The model under review builds one solid part; all positions refer to its coordinate system, in mm. Face numbers are marked on the shaded views. A direction names the side the tool comes from. Give positions to 0.01 mm unless a question says otherwise; leave off trailing zeros. Loops run counter-clockwise (first coordinate to the right, second up) from the corner with the lowest first, then second, coordinate; pieces in that order, holes last. Notation, with made-up numbers: (-35.75, -16) -> (-2.75, -16) arc R19 ccw to (-2.75, 10) -> close; hole circle Ø1 at (5, 57.25). An arc over 180 degrees is marked (long way). Write each question's results on one line, items separated by ' | '. Start each with the question number.
Q1. We need section A-A (z = 20.25). Give the number of separate pieces and of enclosed holes in the cut face, plus the area to 4 significant figures.
Q2. Wall thickness on L1, parallel to Z at x = -28.5, y = -2.5; L2, parallel to X at y = -32, z = 19; L3, parallel to Y at x = 28.5, z = 4: over which ranges is each line inside the solid? List them lowest first. Write a range as [from, to].
Q3. Machinability: for the marked faces 1 and 2, which of the approach directions +Z, -Z, +X, -X, +Y, -Y give a long, thin tool a straight path to every point of the face, cutting with its end or side? Answer none if there is none.
Q4. Insertion check: pin 1 Ø1.3 at (x, z) = (15.5, 12.5) entering from +Y; pin 2 Ø8 at (y, z) = (-31.5, 9.5) entering from -X; pin 3 Ø8 at (x, z) = (-31.5, 9) entering from -Y; pin 4 Ø3 at (x, z) = (-32.5, 19.5) entering from +Y. Each pin has a flat end and moves straight along its axis. Give the tip position at first contact, or say it passes through.
Q5. We need section B-B (x = 0). Write out the cut boundary in (y, z).
Q6. Mouldability with a two-part tool opening along X and no side actions: class the marked faces 3, 4 and 5 as released by +X, released by -X, zero draft, split by the parting line, or undercut.
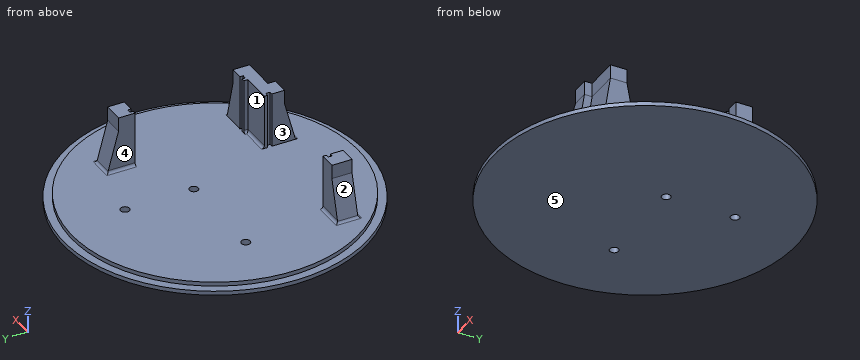
from build123d import *

# Parameters (mm, degrees)
SKIZZE1_R                       = 52
AUFSATZ_LINEAR_AUSTRAGEN1_DEPTH = 3
SKIZZE1_3_R                     = 55
SKIZZE1_3_R_2                   = 52
AUFSATZ_LINEAR_AUSTRAGEN2_DEPTH = 1.5
SKIZZE2_W                       = 5
SKIZZE2_H                       = 4.5
AUFSATZ_LINEAR_AUSTRAGEN5_DEPTH = 20
FASE2_SIZE                      = 4
FASE2_SIZE2                     = 14.92820323
FASE3_SIZE                      = 4
FASE3_SIZE2                     = 14.92820323
VERRUNDUNG1_R                   = 1
SCHNITT_LINEAR_AUSTRAGEN1_REACH = 82.312
SKIZZE3_R                       = 1.6


with BuildPart() as part:
    # Skizze1 → Aufsatz-Linear austragen1 (new body)
    with BuildSketch(Plane.XY):
        Circle(SKIZZE1_R)
    extrude(amount=AUFSATZ_LINEAR_AUSTRAGEN1_DEPTH)

    # Skizze1_3 → Aufsatz-Linear austragen2 (add)
    with BuildSketch(Plane.XY):
        Circle(SKIZZE1_3_R)
        Circle(SKIZZE1_3_R_2, mode=Mode.SUBTRACT)
    extrude(amount=AUFSATZ_LINEAR_AUSTRAGEN2_DEPTH)

    # Skizze2 → Aufsatz-Linear austragen5 (add)
    with BuildSketch(Plane.XY.offset(3)):
        Polygon((21, -33.3), (15, -33.3), (15, -28.7), (16.2, -28.7), (16.2, -27.2), (15, -27.2), (15, -26), (21, -26), align=None)
        with Locations((23.5, -28.25)):
            Rectangle(SKIZZE2_W, SKIZZE2_H)
        Polygon((26, -24.5), (27.2, -24.5), (27.2, -25.7), (28.7, -25.7), (28.7, -24.5), (33.3, -24.5), (33.3, -30.5), (26, -30.5), align=None)
        Polygon((33.3, 21), (33.3, 15), (28.7, 15), (28.7, 16.2), (27.2, 16.2), (27.2, 15), (26, 15), (26, 21), align=None)
        Polygon((-24.5, -26), (-24.5, -27.2), (-25.7, -27.2), (-25.7, -28.7), (-24.5, -28.7), (-24.5, -33.3), (-30.5, -33.3), (-30.5, -26), align=None)
    extrude(amount=AUFSATZ_LINEAR_AUSTRAGEN5_DEPTH)

    # Fase2
    fase2_edges = [part.edges().sort_by_distance(p)[0] for p in [
        (33.3, -27.5, 3),
        (18, -33.3, 3),
        (29.65, 21, 3),
        (-30.5, -29.65, 3),
    ]]
    fase2_side = [part.faces().sort_by_distance(p)[0] for p in [
        (-0.31627578, 0.425239539, 3),
    ]]
    chamfer(fase2_edges, length=FASE2_SIZE, length2=FASE2_SIZE2, reference=fase2_side[0])

    # Fase3
    fase3_edges = [part.edges().sort_by_distance(p)[0] for p in [
        (29.15, -30.5, 3),
        (21, -33.9, 3),
    ]]
    fase3_side = [part.faces().sort_by_distance(p)[0] for p in [
        (-0.466268066, 0.638295482, 3),
    ]]
    chamfer(fase3_edges, length=FASE3_SIZE, length2=FASE3_SIZE2, reference=fase3_side[0])

    # Verrundung1
    verrundung1_edges = [part.edges().sort_by_distance(p)[0] for p in [
        (26, 20, 3),
        (29.65, 25, 3),
        (33.3, 20, 3),
        (-29.5, -33.3, 3),
        (-34.5, -29.65, 3),
        (-29.5, -26, 3),
        (26, -25.25, 3),
        (20.5, -26, 3),
        (37.3, -29.5, 3),
        (31.15, -34.5, 3),
        (25, -35.9, 3),
        (20, -37.3, 3),
    ]]
    fillet(verrundung1_edges, radius=VERRUNDUNG1_R)

    # Skizze3 → Schnitt-Linear austragen1 (cut, up to next)
    with BuildSketch(Plane.XY.offset(3), mode=Mode.PRIVATE) as schnitt_linear_austragen1_sk1:
        with Locations((4.995000167, 4.995918163)):
            Circle(SKIZZE3_R)
    schnitt_linear_austragen1_tool1 = extrude(schnitt_linear_austragen1_sk1.sketch, amount=-SCHNITT_LINEAR_AUSTRAGEN1_REACH, mode=Mode.PRIVATE) & part.part
    # Skizze3 → Schnitt-Linear austragen1 (cut, up to next)
    with BuildSketch(Plane.XY.offset(3), mode=Mode.PRIVATE) as schnitt_linear_austragen1_sk2:
        with Locations((4.995000167, 29.995918163)):
            Circle(SKIZZE3_R)
    schnitt_linear_austragen1_tool2 = extrude(schnitt_linear_austragen1_sk2.sketch, amount=-SCHNITT_LINEAR_AUSTRAGEN1_REACH, mode=Mode.PRIVATE) & part.part
    # Skizze3 → Schnitt-Linear austragen1 (cut, up to next)
    with BuildSketch(Plane.XY.offset(3), mode=Mode.PRIVATE) as schnitt_linear_austragen1_sk3:
        with Locations((-30.004999833, 4.995918163)):
            Circle(SKIZZE3_R)
    schnitt_linear_austragen1_tool3 = extrude(schnitt_linear_austragen1_sk3.sketch, amount=-SCHNITT_LINEAR_AUSTRAGEN1_REACH, mode=Mode.PRIVATE) & part.part
    add(schnitt_linear_austragen1_tool1.solids().sort_by_distance((4.995, 4.995918, 3))[0], mode=Mode.SUBTRACT)
    add(schnitt_linear_austragen1_tool2.solids().sort_by_distance((4.995, 29.995918, 3))[0], mode=Mode.SUBTRACT)
    add(schnitt_linear_austragen1_tool3.solids().sort_by_distance((-30.005, 4.995918, 3))[0], mode=Mode.SUBTRACT)


solid = part.part
Output:
1) separate pieces: 3 | enclosed holes: 0 | area: 190.5 mm2
2) L1: [0, 3] | L2: [-30.5, -24.5], [15, 21] | L3: [-34.23, -25.7], [16.2, 24.73]
3) face 1: +Z, -X, +Y | face 2: +Z, -X, +Y, -Y
4) pin 1: y = -26 | pin 2: x = -33.83 | pin 3: y = -33.3 | pin 4: through
5) outline: (-55, 0) -> (55, 0) -> (55, 1.5) -> (52, 1.5) -> (52, 3) -> (-52, 3) -> (-52, 1.5) -> (-55, 1.5) -> close
6) face 3: undercut | face 4: released by -X | face 5: zero draft
